```python
from build123d import *

# Parameters (mm, degrees)
BOSS_EXTRUDE1_DEPTH = 50.8
SKETCH4_W           = 3.81
SKETCH4_H           = 5.08
BOSS_EXTRUDE5_DEPTH = 50.8
FILLET1_R           = 5.08
FILLET2_SIZE        = 1.27
FILLET2_SIZE_2      = 2.54


with BuildPart() as part:
    # Sketch1 → Boss-Extrude1 (new body)
    with BuildSketch(Plane(origin=(0, 0, 0), x_dir=(0, 0, -1), z_dir=(1, 0, 0))):
        Polygon((0, 0), (106.68, 0), (106.68, 6.35), (68.58, 6.35), (68.58, 44.45), (63.5, 44.45), (63.5, 6.35), (43.18, 6.35), (43.18, 44.45), (38.1, 44.45), (38.1, 6.35), (0, 6.35), align=None)
    extrude(amount=BOSS_EXTRUDE1_DEPTH)

    # Sketch4 → Boss-Extrude5 (add)
    with BuildSketch(Plane(origin=(50.8, 0, 0), x_dir=(0, 0, -1), z_dir=(1, 0, 0))):
        with Locations((61.595, 22.86)):
            Rectangle(SKETCH4_W, SKETCH4_H)
    extrude(amount=-BOSS_EXTRUDE5_DEPTH)

    # Fillet1
    fillet1_edges = [part.edges().sort_by_distance(p)[0] for p in [
        (25.4, 6.35, 0),
        (25.4, 6.35, -38.1),
        (25.4, 6.35, -68.58),
        (25.4, 6.35, -106.68),
    ]]
    fillet(fillet1_edges, radius=FILLET1_R)

    # Fillet2
    # an asymmetric fillet: 2.54, 1.27 mm, written as the material it adds along each edge
    with BuildSketch(Plane(origin=(0, 6.35, -63.5), x_dir=(0, 0, 1), z_dir=(1, 0, 0))) as fillet2_piece_1:
        with BuildLine():
            Bezier((FILLET2_SIZE, 0), (0, 0), (0, -FILLET2_SIZE_2), weights=[1, 0.707106781, 1])
            Line((0, -FILLET2_SIZE_2), (0, 0))
            Line((0, 0), (FILLET2_SIZE, 0))
        make_face()
    extrude(amount=50.8)
    with BuildSketch(Plane(origin=(0, 6.35, -43.18), x_dir=(0, 1, 0), z_dir=(1, 0, 0)), Plane(origin=(50.8, 25.4, -63.5), x_dir=(0, 1, 0), z_dir=(-1, 0, 0))) as fillet2_piece_2:
        with BuildLine():
            Bezier((FILLET2_SIZE_2, 0), (0, 0), (0, -FILLET2_SIZE), weights=[1, 0.707106781, 1])
            Line((0, -FILLET2_SIZE), (0, 0))
            Line((0, 0), (FILLET2_SIZE_2, 0))
        make_face()
    extrude(amount=50.8)
    # an asymmetric fillet: 2.54, 1.27 mm, written as the material it takes off along each edge
    with BuildSketch(Plane(origin=(57.15, 25.4, -59.69), x_dir=(0, 0, -1), z_dir=(-1, 0, 0))) as fillet2_2_piece_1:
        with BuildLine():
            Bezier((FILLET2_SIZE, 0), (0, 0), (0, FILLET2_SIZE_2), weights=[1, 0.707106781, 1])
            Line((0, FILLET2_SIZE_2), (0, 0))
            Line((0, 0), (FILLET2_SIZE, 0))
        make_face()
    extrude(amount=63.5, mode=Mode.SUBTRACT)


solid = part.part
```
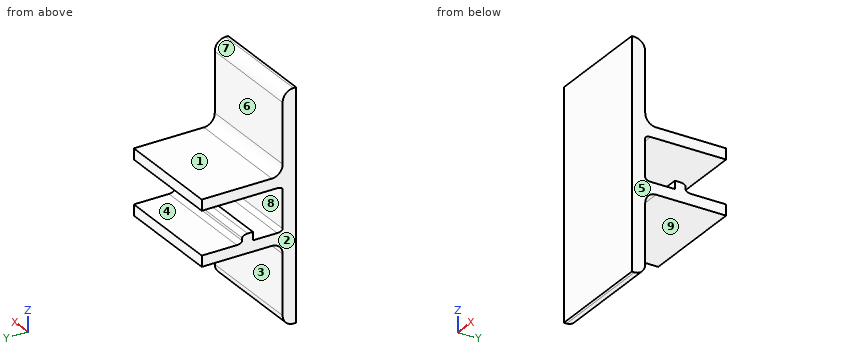
The listing builds one solid part. Answer for the finished solid, in the listing's coordinates (mm). Face numbers are marked on the shaded views. A direction names the side the tool comes from. Coordinates: 2 decimals unless noted, no trailing zeros. Order: outer loops, then holes, each group sorted by start corner. A loop starts at its lowest first (then second) coordinate and runs counter-clockwise, first axis right, second up. Notation, with made-up numbers: M 81,8 L 109,8 A27 cw 109,26 Z; hole C 40.25,-9.5 d6. An arc over 180 degrees is marked long. Answer as a JSON object with one key per item and string values. Group by question number.
1. Flat-ended cylindrical pins translate along their axes: P1, Ø10, axis at x = 22.5, y = 26.5, coming from the +Z side; P2, Ø5, axis at x = 11.5, y = 37.5, coming from the -Z side; P3, Ø5, axis at x = 39.5, y = 12, coming from the +Z side. Find the tip coordinate at first contact, or state that the pin passes through.
2. Determine the mould class of the marked faces 6, 7, 8 and 9 for opening direction Z: released by +Z, released by -Z, zero draft, split by the parting line, or undercut.
3. Straight lines are drawn through the part: line 1 (Z direction, x = 5, y = 33); line 2 (Z direction, x = 3.5, y = 22.5); line 3 (Y direction, x = 6, z = -47.5). For each, find the intervals that lie inside material, in ascending order.
4. Section B-B on z = -98.5 is taken. Write down the section's boundary in (x, y).
5. A tool of negligible diameter and unlimited length cuts with its end or side. For the marked faces 1, 2, 3, 4 and 5, from which of +Z, -Z, +X, -X, +Y, -Y can it reach the whole face along a straight path? Write none if from no direction.
6. Section A-A on y = 35.5 is taken. Write down the section's boundary in (x, z).
Values follow:
{
 "1": {"P1": "z = -38.1", "P2": "z = -68.58", "P3": "z = -37.72"},
 "2": {"face 6": "zero draft", "face 7": "released by +Z", "face 8": "undercut", "face 9": "released by -Z"},
 "3": {"line 1": "-68.58 to -63.5, -43.18 to -38.1", "line 2": "-68.58 to -59.69, -43.18 to -38.1", "line 3": "0 to 6.35"},
 "4": {"outline": "M 0,0 L 50.8,0 L 50.8,6.35 L 0,6.35 Z"},
 "5": {"face 1": "+Z, +X, -X, +Y", "face 2": "+Z, -Z, -X, +Y, -Y", "face 3": "-Z, +X, -X, +Y", "face 4": "+X, -X, +Y", "face 5": "+Z, -Z, +X, +Y, -Y"},
 "6": {"outline": "M 0,-68.58 L 50.8,-68.58 L 50.8,-63.5 L 0,-63.5 Z; M 0,-43.18 L 50.8,-43.18 L 50.8,-38.1 L 0,-38.1 Z"}
}
